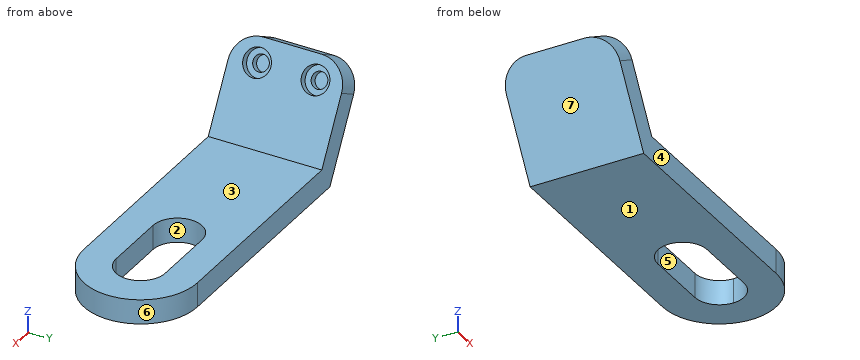
from build123d import *

# Parameters (mm, degrees)
F1_DEPTH = 44.704
F3_DEPTH = 9.652
F4_DEPTH = 25.4
F5_R     = 10.922
F6_R     = 5.461
F6_R_2   = 3.175
F7_DEPTH = 3.175
F8_DEPTH = 6.35


with BuildPart() as f1:
    # F0 (on Front) → F1 (new body)
    with BuildSketch(Plane.XZ):
        Polygon((-5.5725847982, 0), (85.852, 0), (85.852, 9.652), (0, 9.652), (-19.05, 42.6475678842), (-27.4088771973, 37.8215678842), align=None)
    extrude(amount=F1_DEPTH)

    # F2 (on face) → F3 (join)
    with BuildSketch(Plane.XY.offset(9.652)):
        with BuildLine():
            ThreePointArc((85.852, -12.7), (92.676994652, -15.527005348), (95.504, -22.352))
            ThreePointArc((95.504, -22.352), (92.676994652, -29.176994652), (85.852, -32.004))
            Line((85.852, -32.004), (85.852, -44.704))
            ThreePointArc((85.852, -44.704), (108.204, -22.352), (85.852, 0))
            Line((85.852, 0), (85.852, -12.7))
        make_face()
    extrude(amount=-F3_DEPTH)

    # F2 (on face) → F4 (cut)
    with BuildSketch(Plane.XY.offset(9.652)):
        with BuildLine():
            ThreePointArc((85.852, -32.004), (92.676994652, -29.176994652), (95.504, -22.352))
            ThreePointArc((95.504, -22.352), (92.676994652, -15.527005348), (85.852, -12.7))
            ThreePointArc((85.852, -12.7), (76.2, -22.352), (85.852, -32.004))
        make_face()
        with BuildLine():
            ThreePointArc((85.852, -32.004), (76.2, -22.352), (85.852, -12.7))
            Line((85.852, -12.7), (60.452, -12.7))
            ThreePointArc((60.452, -12.7), (67.276994652, -15.527005348), (70.104, -22.352))
            ThreePointArc((70.104, -22.352), (67.276994652, -29.176994652), (60.452, -32.004))
            Line((60.452, -32.004), (85.852, -32.004))
        make_face()
        with BuildLine():
            ThreePointArc((70.104, -22.352), (67.276994652, -15.527005348), (60.452, -12.7))
            ThreePointArc((60.452, -12.7), (50.8, -22.352), (60.452, -32.004))
            ThreePointArc((60.452, -32.004), (67.276994652, -29.176994652), (70.104, -22.352))
        make_face()
    extrude(amount=-F4_DEPTH, mode=Mode.SUBTRACT)

    # F5
    f5_edges = [f1.edges().sort_by_distance(p)[0] for p in [
        (-23.229439, -44.704, 40.234568),
        (-23.229439, 0, 40.234568),
    ]]
    fillet(f5_edges, radius=F5_R)

    # F6 (on face) → F7 (cut)
    with BuildSketch(Plane(origin=(4.1794385987, 0, 2.413), x_dir=(0, 1, 0), z_dir=(0.8660254038, 0, 0.5))):
        with Locations((-33.782, 37.3698046379)):
            Circle(F6_R)
        with Locations((-33.782, 37.3698046379)):
            Circle(F6_R_2, mode=Mode.SUBTRACT)
        with Locations((-10.7671008632, 37.3698046379)):
            Circle(F6_R)
        with Locations((-10.7671008632, 37.3698046379)):
            Circle(F6_R_2, mode=Mode.SUBTRACT)
    extrude(amount=-F7_DEPTH, mode=Mode.SUBTRACT)

    # F8 (cut): faces of the model
    f8_faces = [f1.faces().sort_by_distance(p)[0] for p in [
        (-14.5054637203, -33.782, 34.7762001509),
        (-14.5054637203, -10.7671008632, 34.7762001509),
    ]]
    extrude(f8_faces, amount=-F8_DEPTH, mode=Mode.SUBTRACT)


solid = f1.part
Here's how the part is built. I have some questions about the finished solid (model axes, mm). Face numbers are marked on the shaded views. A direction names the side the tool comes from. Round coordinates to 2 decimals unless told otherwise and drop trailing zeros. Loops run counter-clockwise (first coordinate to the right, second up) from the corner with the lowest first, then second, coordinate; pieces in that order, holes last. Notation, with made-up numbers: (66, -4) - (77, -4) arc R24 ccw to (77, 31) - close; hole circle Ø10 at (84, 43.5). An arc over 180 degrees is marked (long way). One line per question, with ' | ' between items. Start each with the question number.
Q1. I want a section at C-C (z = 8). Write out the boundary of the cut face in (x, y).
Q2. We'd pull the mould along X, two halves only. Please class the marked faces 4, 5, 6 and 7: +X half, -X half, draft (parallel to the pull), parting line (faces both ways), or undercut.
Q3. I want a section at B-B (y = -21). Write out the boundary of the cut face in (x, z), then the cut area to 3 significant figures.
Q4. Please list where these lines run through material, in increasing order: line 1 (Y direction, x = 64.5, z = 7); line 2 (Z direction, x = 13.5, y = -31); line 3 (X direction, y = -7.5, z = 29.5). Write a range as [from, to].
Q5. I want a section at A-A (x = 64). Write out the boundary of the cut face in (y, z).
Q6. I want a section at D-D (y = -41.5). Write out the boundary of the cut face in (x, z).
Q7. Will these pins go through, and if not, where does the flat tip stop? pin 1 (3 mm diameter, centred on y = -25, z = 36, fed in from -X); pin 2 (3 mm diameter, centred on y = -23.5, z = 14, fed in from +X); pin 3 (8 mm diameter, centred on x = 93, y = -31, fed in from +Z); pin 4 (4 mm diameter, centred on x = 17.5, y = -32, fed in from -Z).
Q8. For the marked faces 1, 2 and 3, which set-ups out of +Z, -Z, +X, -X, +Y, -Y let a thin tool reach every point of the face, with its end or its side?
Response values:
1) outline: (-10.19, -44.7) - (85.85, -44.7) arc R22.35 ccw to (85.85, 0) - (-10.19, 0) - close; hole (60.45, -32) - (85.85, -32) arc R9.65 ccw to (85.85, -12.7) - (60.45, -12.7) arc R9.65 ccw to start
2) face 4: draft | face 5: undercut | face 6: +X half | face 7: -X half
3) outline: (-27.41, 37.82) - (-5.57, 0) - (50.9, 0) - (50.9, 9.65) - (0, 9.65) - (-19.05, 42.65) - close; (95.41, 0) - (108.16, 0) - (108.16, 9.65) - (95.41, 9.65) - close | area: 1,040 mm²
4) line 1: y = [-44.7, -32], [-12.7, 0] | line 2: z = [0, 9.65] | line 3: x = [-22.6, -15.13], [-14.89, -11.46]
5) outline: (-44.7, 0) - (-32, 0) - (-32, 9.65) - (-44.7, 9.65) - close; (-12.7, 0) - (0, 0) - (0, 9.65) - (-12.7, 9.65) - close
6) outline: (-25.81, 35.06) - (-5.57, 0) - (97.38, 0) - (97.38, 9.65) - (0, 9.65) - (-17.45, 39.88) - close
7) pin 1: stops at x = -27.22 | pin 2: stops at x = -1.64 | pin 3: stops at z = 9.65 | pin 4: stops at z = 0
8) face 1: -Z, +X, -X, +Y, -Y | face 2: +Z, -Z | face 3: +Z, +X, +Y, -Y
